Work out the finished part from the listing and answer in its coordinate system (mm). A direction names the side the tool comes from. Give positions to 0.01 mm unless a question says otherwise; leave off trailing zeros. Order: outer loops, then holes, each group sorted by start corner. A loop starts at its lowest first (then second) coordinate and runs counter-clockwise, first axis right, second up. Notation, with made-up numbers: (-10, -27) - (25, -27) arc R30 cw to (25, 6) - close; hole circle Ø11 at (29.5, 9.5). An arc over 180 degrees is marked (long way). Put each result on its own line as item: value.
Autodesk Inventor part; units mm, degrees
ref_plane "YZ Plane" through (0, 0, 0) normal (1, 0, 0) x (0, 1, 0)
ref_plane "XZ Plane" through (0, 0, 0) normal (0, 1, 0) x (-1, 0, 0)
ref_plane "XY Plane" through (0, 0, 0) normal (0, 0, 1) x (1, 0, 0)
sketch "Sketch1" plane through (0, 0, 0) normal (1, 0, 0) x (0, 1, 0)
  line L0 (0, 61) -> (3, 61)
  line L1 (3, 61) -> (3, 44.8)
  line L2 (3, 44.8) -> (10, 44.8)
  line L3 (10, 44.8) -> (10, 41.8)
  line L4 (10, 41.8) -> (16, 41.8)
  line L5 (16, 41.8) -> (16, 35.8)
  line L6 (16, 35.8) -> (15.99, 35.8)
  line L7 (15.99, 35.8) -> (15.99, 6)
  line L8 (15.99, 6) -> (16, 6)
  line L9 (16, 6) -> (16, 0)
  line L10 (16, 0) -> (0, 0)
  line L11 (0, 0) -> (0, 61)
  line L12 (5.75, 45.4) -> (3, 45.4)
  line L13 (3, 45.4) -> (3, 44.8)
  line L14 (3, 44.8) -> (5.75, 44.8)
  line L15 (5.75, 44.8) -> (5.75, 45.4)
  point P0 (1.5, 61)
  dimension "d0" = 6
  dimension "d1" = 32
  dimension "d2" = 6
  dimension "d3" = 19.2
  dimension "d4" = 41.8
  dimension "d5" = 3
  dimension "d6" = 20
  dimension "d7" = 0.01
  dimension "d24" = 0.6
  dimension "d25" = 11.5
revolve "Revolution1" add sketch "Sketch1" angle 360 about axis through (0, 0, 0) along (0, 0, 1)
sketch "Sketch2" plane through (0, 0, 61) normal (0, 0, 1) x (1, 0, 0)
  arc A0 (1.6583, 2.5) -> (-1.6583, 2.5) centre (0, 0) ccw
  line L0 (-1.6583, 2.5) -> (1.6583, 2.5)
  circle A1 centre (0, 0) radius 3
  dimension "d9" = 2.5
extrude "Extrusion1" cut sketch "Sketch2" against normal blind 12 contours L0 A0
sketch "Sketch3" plane through (0, 0, 44.8) normal (0, 0, 1) x (1, 0, 0)
  line L0 (-9, 4.3589) -> (-9, -4.3589)
  line L1 (9, 4.3589) -> (9, -4.3589)
  arc A0 (-9, 4.3589) -> (-9, -4.3589) centre (0, 0) ccw
  arc A1 (9, -4.3589) -> (9, 4.3589) centre (0, 0) ccw
  circle A2 centre (0, 0) radius 10 construction
  dimension "d12" = 18
extrude "Extrusion2" cut sketch "Sketch3" against normal up to surface (3 mm away)
sketch "Sketch4" plane through (0, 0, 41.8) normal (0, 0, 1) x (1, 0, 0)
  line L0 (0, 0) -> (-9.1924, 9.1924) construction
  circle A0 centre (-9.1924, 9.1924) radius 1.5
  line L1 (0, 0) -> (-13, 0) construction
  circle A1 centre (-9.1924, -9.1924) radius 1.5
  circle A2 centre (9.1924, -9.1924) radius 1.5
  circle A3 centre (9.1924, 9.1924) radius 1.5
  dimension "d15" = 3
  dimension "d16" = 13
  dimension "d17" = 45
  dimension "d20" = 360
extrude "Extrusion3" cut sketch "Sketch4" against normal blind 6
properties part number "PlanetaryGearbox"
(1) Straight lines are drawn through the part: line 1 (Z direction, x = -7.5, y = 12.5); line 2 (Z direction, x = -5.5, y = 0); line 3 (Y direction, x = -3.5, z = 16). For each, find the intervals that lie inside material, in ascending order.
Geometry check:
line 1: z = 0 to 41.8
line 2: z = 0 to 45.4
line 3: y = -15.6 to 15.6
(2) Determine the mould class of faces 6 (the face through (9, -9, 35.8)), 7 (the face through (2.5, 2.5, 45.4)), 8 (the face through (0, 2.5, 55)) for opening direction Y: pulls with the +Y half, pulls with the -Y half, needs draft (parallel to the pull), parting line crosses it, or undercut.
Geometry check:
face 6: undercut
face 7: needs draft
face 8: pulls with the +Y half
(3) Given pin 1 (1.8 mm diameter, centred on x = -9.19, y = -9.19, fed in from +Z); pin 2 (3.5 mm diameter, centred on y = -0.5, z = 44, fed in from -X); pin 3 (1.5 mm diameter, centred on y = 1.5, z = 43.5, fed in from +X); pin 4 (8 mm diameter, centred on x = -5, y = 6, fed in from -Z), each flat-ended and moving along its own axis, determine where each tip first touches the part or whether it passes through.
Geometry check:
pin 1: stops at z = 35.8
pin 2: stops at x = -9
pin 3: stops at x = 9
pin 4: stops at z = 0
(4) Section C-C, the plane z = 22 is taken. Write down the section's boundary in (x, y), then the cut area to 3 significant figures.
Geometry check:
outline: circle Ø31.98 at (0, 0)
area: 803 mm²
(5) A tool of negligible diameter and unlimited length cuts with its end or side. For faces 1 (the face through (0, 0, 61)), 2 (the face through (-15.62, -3.47, 38.76)), 3 (the face through (9, 0, 43)), 4 (the face through (-9, 0, 43)), 5 (the face through (10, 0, 41.8)), from which of +Z, -Z, +X, -X, +Y, -Y can it reach the whole face along a straight path? Write none if from no direction.
Geometry check:
face 1: +Z, +X, -X, +Y, -Y
face 2: +Z, -Z
face 3: +Z, +X, +Y, -Y
face 4: +Z, -X, +Y, -Y
face 5: +Z
